Design review of the part built by this model. Coordinates are the model's own, in mm. Give positions to 0.01 mm unless a question says otherwise; leave off trailing zeros. Loops run counter-clockwise (first coordinate to the right, second up) from the corner with the lowest first, then second, coordinate; pieces in that order, holes last. Notation, with made-up numbers: M 17.25,48.5 L 68.25,48.5 A17 ccw 68.25,70.5 Z; hole C -36.75,36 d7. An arc over 180 degrees is marked long. Use a Markdown table: item, result. Add a question column.
(1) Draft analysis for pull direction Y (two halves, no side actions). For faces 1 (the face through (39, 0, 0)), 2 (the face through (96, 0, 3)), 3 (the face through (5.19, -9.98, 3.45)), state which applies: pulls with the +Y half, pulls with the -Y half, needs draft (parallel to the pull), parting line crosses it, or undercut.
(2) Add section A-A, the plane y = 7. Give the boundary of the cut face in (x, z).
(3) For probe 1 along Y at (x, z) = (0, 2.25); probe 2 along X at (y, z) = (-1.5, 3.25); probe 3 along Y at (x, z) = (50, 4.5), list the stretches that pass through material, from the lowest coordinate up.
(4) Insertion check: pin 1 Ø3 at (x, y) = (30, 0) entering from +Z; pin 2 Ø6 at (x, y) = (50, 0) entering from +Z; pin 3 Ø3 at (y, z) = (7, 2.5) entering from +X (3 decimals); pin 4 Ø4 at (y, z) = (-5.5, 2.5) entering from +X. Each pin has a flat end and moves straight along its axis. Give the tip position at first contact, or say it passes through.
(5) Add section B-B, the plane z = 2. State how many separate pieces and enclosed holes the cut face has, then the cut area to 3 significant figures.
```python
from build123d import *

# Parameters (mm, degrees)
ESQUISSE1_R             = 11.25
BOSS_EXTRU_1_DEPTH      = 7
ESQUISSE2_R             = 1.8
ENL_V_MAT_EXTRU_1_DEPTH = 10


with BuildPart() as part:
    # Esquisse1 → Boss.-Extru.1 (new body)
    with BuildSketch(Plane.XY):
        with BuildLine():
            ThreePointArc((0, 16), (-16, 0), (0, -16))
            add(Edge.make_bspline(
                [(0, -16), (40, 0), (80, -16)],
                knots=[0, 0, 0, 1, 1, 1], degree=2))
            ThreePointArc((80, -16), (96, 0), (80, 16))
            add(Edge.make_bspline(
                [(0, 16), (40, 0), (80, 16)],
                knots=[0, 0, 0, 1, 1, 1], degree=2))
        make_face()
        with Locations((80, 0)):
            Circle(ESQUISSE1_R, mode=Mode.SUBTRACT)
        Circle(ESQUISSE1_R, mode=Mode.SUBTRACT)
    extrude(amount=BOSS_EXTRU_1_DEPTH)

    # Esquisse2 → Enlèv. mat.-Extru.1 (cut)
    with BuildSketch(Plane.XY.offset(7)):
        with Locations((30, 0)):
            Circle(ESQUISSE2_R)
        with Locations((50, 0)):
            Circle(ESQUISSE2_R)
    extrude(amount=-ENL_V_MAT_EXTRU_1_DEPTH, mode=Mode.SUBTRACT)


solid = part.part
```
Established:
| question | item | result |
|---|---|---|
| 1 | face 1 | needs draft |
| 1 | face 2 | parting line crosses it |
| 1 | face 3 | undercut |
| 2 | outline | M -14.39,0 L -8.81,0 L -8.81,7 L -14.39,7 Z; M 8.81,0 L 71.19,0 L 71.19,7 L 8.81,7 Z; M 88.81,0 L 94.39,0 L 94.39,7 L 88.81,7 Z |
| 3 | probe 1 | -16 to -11.25, 11.25 to 16 |
| 3 | probe 2 | -15.93 to -11.15, 11.15 to 29.01, 30.99 to 49.01, 50.99 to 68.85, 91.15 to 95.93 |
| 3 | probe 3 | -8.5 to -1.8, 1.8 to 8.5 |
| 4 | pin 1 | through |
| 4 | pin 2 | z = 7 |
| 4 | pin 3 | x = 95.025 |
| 4 | pin 4 | x = 95.61 |
| 5 | separate pieces | 1 |
| 5 | enclosed holes | 4 |
| 5 | area | 1,700 mm^2 |
